```python
from build123d import *

# Parameters (mm, degrees)
SKETCH1_W           = 6.1976
SKETCH1_H           = 6.1976
BOSS_EXTRUDE1_DEPTH = 3.5052
SKETCH2_R           = 1.7526
BOSS_EXTRUDE2_DEPTH = 9.4996


with BuildPart() as part:
    # Sketch1 → Boss-Extrude1 (new body)
    with BuildSketch(Plane.XY):
        Rectangle(SKETCH1_W, SKETCH1_H)
    extrude(amount=-BOSS_EXTRUDE1_DEPTH)

    # Sketch2 → Boss-Extrude2 (add)
    with BuildSketch(Plane.XY):
        Circle(SKETCH2_R)
    extrude(amount=BOSS_EXTRUDE2_DEPTH)


solid = part.part
```
Source: CAD feature listing. Evaluate the final solid. Frame: model axes, mm. A direction names the side the tool comes from. Round coordinates to 2 decimals unless told otherwise and drop trailing zeros. Loops run counter-clockwise (first coordinate to the right, second up) from the corner with the lowest first, then second, coordinate; pieces in that order, holes last.
(1) Section query D-D (y = -2.25). Output: boundary loops of the cut face in (x, z), and give its area (3 significant figures).
From the geometry:
outline: (-3.1, -3.51) - (3.1, -3.51) - (3.1, 0) - (-3.1, 0) - close
area: 21.7 mm2
(2) Section query A-A (x = 0). Output: boundary loops of the cut face in (y, z).
From the geometry:
outline: (-3.1, -3.51) - (3.1, -3.51) - (3.1, 0) - (1.75, 0) - (1.75, 9.5) - (-1.75, 9.5) - (-1.75, 0) - (-3.1, 0) - close
(3) Access query for faces 1 (the flat face through (0, 3.099, -2)), 2 (the flat face through (-1.4, -1.3, 0)). Directions: +Z, -Z, +X, -X, +Y, -Y. A direction counts if a zero-diameter tool reaches every point of the face in a straight line with its end or side. Return the directions, or none.
From the geometry:
face 1: +Z, -Z, +X, -X, +Y
face 2: +Z
(4) Material intervals for probe 1 along Z at (x, y) = (-2, -1); probe 2 along X at (y, z) = (0.25, 5.5); probe 3 along Y at (x, z) = (1.5, 1.75), sorted ascending.
From the geometry:
probe 1: z = -3.51 to 0
probe 2: x = -1.73 to 1.73
probe 3: y = -0.91 to 0.91
(5) Section query C-C (z = 3.75). Output: boundary loops of the cut face in (x, y).
From the geometry:
outline: circle Ø3.51 at (0, 0)
